Design review of the part shown in the three views and the two pictorial views. Dimensions are in mm from the part's minimum x, y and z. A direction names the side the tool comes from. Give positions to 0.01 mm unless a question says otherwise; leave off trailing zeros. Loops run counter-clockwise (first coordinate to the right, second up) from the corner with the lowest first, then second, coordinate; pieces in that order, holes last.
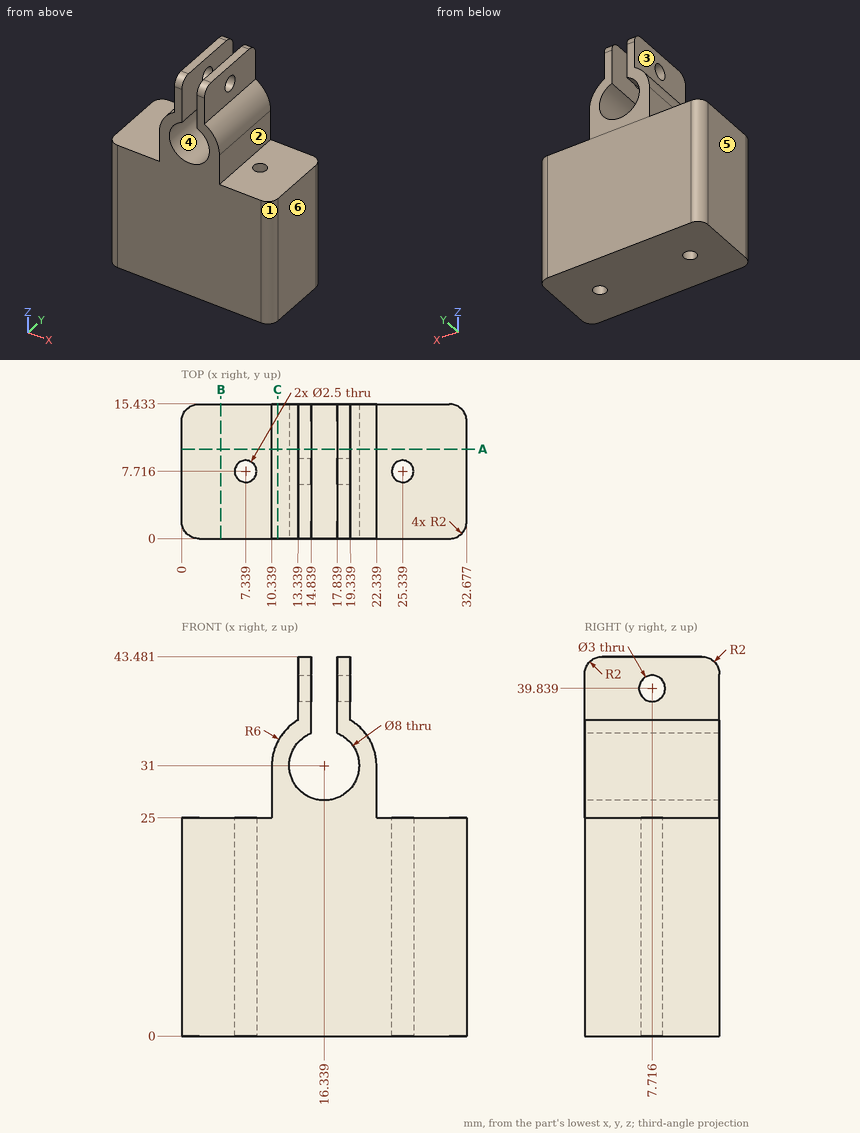
Q1. Take a section at C-C (x = 11). Give the boundary of the cut face in (y, z).
Results:
outline: (0, 0) - (15.43, 0) - (15.43, 33.74) - (0, 33.74) - close
Q2. Take a section at B-B (x = 4.5). Give the boundary of the cut face in (y, z), plus the area to 3 significant figures.
Results:
outline: (0, 0) - (15.43, 0) - (15.43, 25) - (0, 25) - close
area: 386 mm2
Q3. Insertion check: pin 1 (2 mm diameter, centred on y = 5.5, z = 41.5, fed in from -X); pin 2 (2 mm diameter, centred on y = 7.5, z = 39.5, fed in from +X); pin 3 (5 mm diameter, centred on x = 5.5, y = 9, fed in from +Z); pin 4 (5 mm diameter, centred on y = 6, z = 28.5, fed in from +X). Each pin has a flat end and moves straight along its axis. Give the tip position at first contact, or say it passes through.
Results:
pin 1: stops at x = 13.34
pin 2: passes through
pin 3: stops at z = 25
pin 4: stops at x = 22.34
Q4. Wall thickness on line 1 (Y direction, x = 7.5, z = 23.5) (1 decimal); line 2 (Z direction, x = 28, y = 7); line 3 (X direction, y = 9.75, z = 31): over which ranges is each line inside the solid? List them lowest first.
Results:
line 1: y = 0 to 6.5, 9 to 15.4
line 2: z = 0 to 25
line 3: x = 10.34 to 12.34, 20.34 to 22.34
Q5. Draft analysis for pull direction X (two halves, no side actions). For the marked faces 4, 5 and 6, state which applies: pulls with the +X half, pulls with the -X half, needs draft (parallel to the pull), parting line crosses it, or undercut.
Results:
face 4: undercut
face 5: pulls with the -X half
face 6: pulls with the +X half
Q6. Tool access review of the marked faces 1, 2 and 3: name each direction out of +Z, -Z, +X, -X, +Y, -Y from which nothing blocks a thin tool from reaching the whole face with its end or side.
Results:
face 1: +Z, -Z, +X, -Y
face 2: +Z, +X, +Y, -Y
face 3: +Z, -X, +Y, -Y
Q7. Take a section at A-A (y = 10.25). Give the boundary of the cut face in (x, z).
Results:
outline: (0, 0) - (32.68, 0) - (32.68, 25) - (22.34, 25) - (22.34, 31) arc R6 ccw to (19.34, 36.2) - (19.34, 43.48) - (17.84, 43.48) - (17.84, 34.71) arc R4 cw (long way) to (14.84, 34.71) - (14.84, 43.48) - (13.34, 43.48) - (13.34, 36.2) arc R6 ccw to (10.34, 31) - (10.34, 25) - (0, 25) - close
